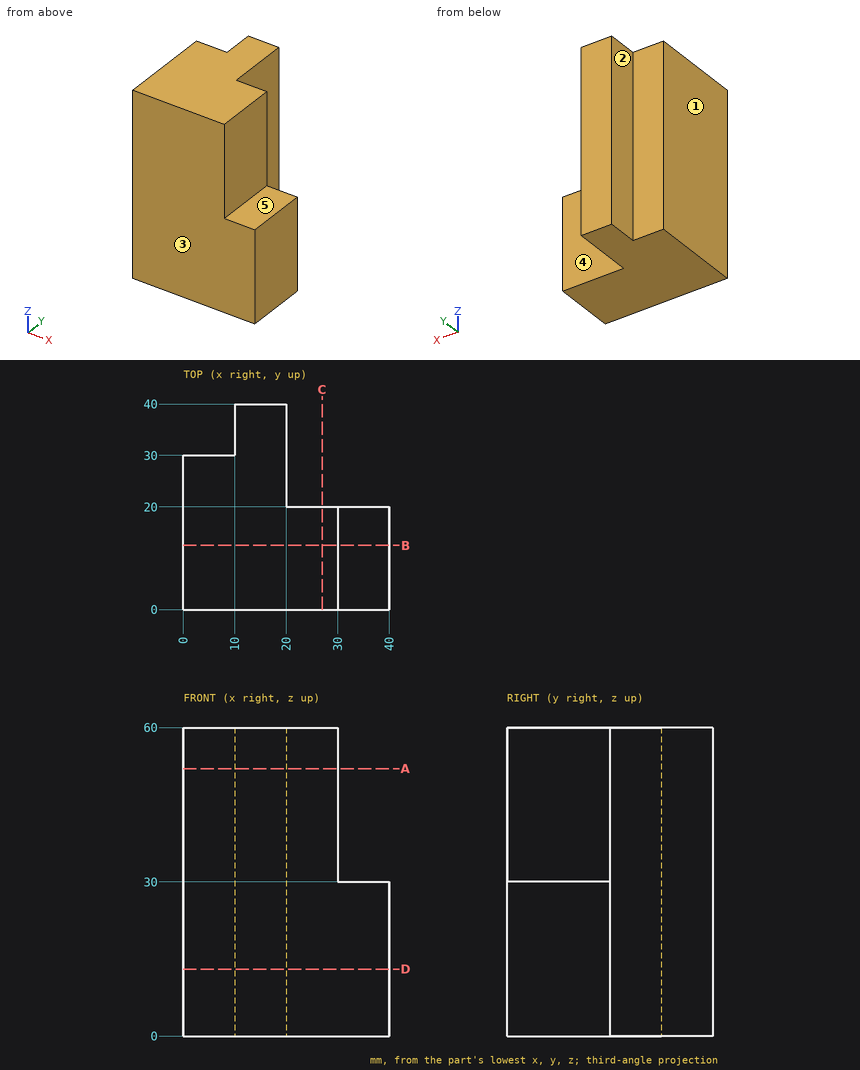
Here's the drawing with two shaded views (mm, measured from the low corner). I have some questions. A direction names the side the tool comes from. Coordinates: 2 decimals unless noted, no trailing zeros. Write each loop counter-clockwise with the first axis right and the second up, starting at its lowest first coordinate (ties: lowest second). Pieces come first, ordered by that corner, then holes. Notation, with made-up numbers: M 7,66 L 43,66 A17 cw 43,73 Z; hole C 69.5,64 d6. An arc over 180 degrees is marked long. Use one line per item in the form item = value.
Q1. For the marked faces 1, 2, 3, 4 and 5, which set-ups out of +Z, -Z, +X, -X, +Y, -Y let a thin tool reach every point of the face, with its end or its side?
Model answer:
face_1 = +Z, -Z, -X, +Y, -Y
face_2 = +Z, -Z, -X, +Y
face_3 = +Z, -Z, +X, -X, -Y
face_4 = +Z, -Z, +X, +Y
face_5 = +Z, +X, +Y, -Y
Q2. If we section it at C-C (x = 27): Write out the boundary of the cut face in (y, z).
Model answer:
outline = M 0,0 L 20,0 L 20,60 L 0,60 Z
Q3. If we section it at D-D (z = 13): Write out the boundary of the cut face in (x, y).
Model answer:
outline = M 0,0 L 40,0 L 40,20 L 20,20 L 20,40 L 10,40 L 10,30 L 0,30 Z
Q4. If we section it at A-A (z = 52): Write out the boundary of the cut face in (x, y), then the cut area to 3 significant figures.
Model answer:
outline = M 0,0 L 30,0 L 30,20 L 20,20 L 20,40 L 10,40 L 10,30 L 0,30 Z
area = 900 mm^2
Q5. I need wall thicknesses on line 1 along Y through (x, z) = (28.5, 33.5); line 2 along Z through (x, y) = (32.5, 10). Which ranges of each line are inside material? Lowest first, please. Write a range as from..to.
Model answer:
line_1 = 0..20
line_2 = 0..30
Q6. For P1, Ø12, axis at x = 10.5, z = 12.5, coming from the -Y side; P2, Ø22, axis at y = 32.5, z = 32.5, coming from the +X side; P3, Ø10, axis at x = 27, z = 36.5, coming from the +Y side; P4, Ø8, axis at x = 3, z = 15.5, coming from the +Y side, each with a flat end and sliding along its axis, tell me the tip position at first contact or that it passes through.
Model answer:
P1 = 0
P2 = 20
P3 = 20
P4 = 30
Q7. If we section it at B-B (y = 12.5): Write out the boundary of the cut face in (x, z), then the cut area to 3 significant figures.
Model answer:
outline = M 0,0 L 40,0 L 40,30 L 30,30 L 30,60 L 0,60 Z
area = 2,100 mm^2
